Could you check a few things on this model? Use its own coordinates, in mm. A direction names the side the tool comes from. Coordinates: 2 decimals unless noted, no trailing zeros. Write each loop counter-clockwise with the first axis right and the second up, starting at its lowest first coordinate (ties: lowest second). Pieces come first, ordered by that corner, then holes. Notation, with made-up numbers: M 86.25,-22 L 134.25,-22 A29 cw 134.25,8 Z; hole C 66,59 d10. An arc over 180 degrees is marked long. Write item = value, one per line.
```python
from build123d import *

# Parameters (mm, degrees)
SKETCH1_R           = 2.54
BOSS_EXTRUDE1_DEPTH = 3.175


with BuildPart() as part:
    # Sketch1 → Boss-Extrude1 (new body)
    with BuildSketch(Plane.XY):
        with BuildLine():
            Line((-9.982299112, -2.937462922), (-4.078000987, -12.791080219))
            ThreePointArc((-4.078000987, -12.791080219), (-3.40491243, -14.361697822), (-3.175, -16.05492791))
            Line((-3.175, -16.05492791), (-3.175, -35.993911504))
            Line((-3.175, -35.993911504), (3.175, -35.993911504))
            Line((3.175, -35.993911504), (3.175, -16.05492791))
            ThreePointArc((3.175, -16.05492791), (3.40491243, -14.361697822), (4.078000987, -12.791080219))
            Line((4.078000987, -12.791080219), (9.982299112, -2.937462922))
            ThreePointArc((9.982299112, -2.937462922), (8.865013598, 4.281926793), (1.563076923, 4.504717202))
            ThreePointArc((1.563076923, 4.504717202), (0, 3.966813736), (-1.563076923, 4.504717202))
            ThreePointArc((-1.563076923, 4.504717202), (-8.865013598, 4.281926793), (-9.982299112, -2.937462922))
        make_face()
        with Locations((5.08, 0)):
            Circle(SKETCH1_R, mode=Mode.SUBTRACT)
        with Locations((-5.08, 0)):
            Circle(SKETCH1_R, mode=Mode.SUBTRACT)
    extrude(amount=BOSS_EXTRUDE1_DEPTH)


solid = part.part
```
Item 1: Imagine slicing it at B-B (z = 2.1). Write out the boundary of the cut face in (x, y) (3 decimals), and give its area (3 significant figures).
Numbers:
outline = M -9.982,-2.937 L -4.078,-12.791 A6.35 cw -3.175,-16.055 L -3.175,-35.994 L 3.175,-35.994 L 3.175,-16.055 A6.35 cw 4.078,-12.791 L 9.982,-2.937 A5.715 ccw 1.563,4.505 A2.54 cw -1.563,4.505 A5.715 ccw Z; hole C -5.08,0 d5.08; hole C 5.08,0 d5.08
area = 411 mm²
Item 2: Imagine slicing it at C-C (x = -5.08). Write out the boundary of the cut face in (y, z) (3 decimals), and give its area (3 significant figures).
Numbers:
outline = M -11.119,0 L -2.54,0 L -2.54,3.175 L -11.119,3.175 Z; M 2.54,0 L 5.715,0 L 5.715,3.175 L 2.54,3.175 Z
area = 37.3 mm²
Item 3: Imagine slicing it at A-A (y = 0). Write out the boundary of the cut face in (x, z) (3 decimals), and give its area (3 significant figures).
Numbers:
outline = M -10.795,0 L -7.62,0 L -7.62,3.175 L -10.795,3.175 Z; M -2.54,0 L 2.54,0 L 2.54,3.175 L -2.54,3.175 Z; M 7.62,0 L 10.795,0 L 10.795,3.175 L 7.62,3.175 Z
area = 36.3 mm²
Item 4: If we mould it in two halves opening along X, with no side actions, what happens to faces 4 (the face through (0, -35.994, 2)), 5 (the face through (8.947, 4.208, 1.565)), 6 (the face through (-3.41, -14.34, 1.57))? For each: pulls with the +X half, pulls with the -X half, needs draft (parallel to the pull), parting line crosses it, or undercut.
Numbers:
face_4 = needs draft
face_5 = undercut
face_6 = pulls with the -X half
Item 5: Imagine slicing it at D-D (y = -18). Write out the boundary of the cut face in (x, z) (3 decimals).
Numbers:
outline = M -3.175,0 L 3.175,0 L 3.175,3.175 L -3.175,3.175 Z
Item 6: For faces 1 (the face through (-3.175, -26, 2)), 2 (the face through (0.024, 3.967, 1.565)), 3 (the face through (3.175, -26, 2)), which set-ups out of +Z, -Z, +X, -X, +Y, -Y let a thin tool reach every point of the face, with its end or its side?
Numbers:
face_1 = +Z, -Z, -X, -Y
face_2 = +Z, -Z, +Y
face_3 = +Z, -Z, +X, -Y
Item 7: I'm going to push flat-ended pins straight in: P1, Ø4, axis at x = 5.08, y = 0, coming from the -Z side; P2, Ø1, axis at y = -29, z = 2, coming from the -X side (3 decimals); P3, Ø1, axis at x = 6, z = 1.5, coming from the -Y side; P4, Ø1.6, axis at y = -24, z = 1.5, coming from the +X side (3 decimals). Where does each tip first touch, or does it pass through?
Numbers:
P1 = through
P2 = -3.175
P3 = -10.42
P4 = 3.175
Item 8: If I drill on line 1 along Y through (x, z) = (4, 1.95); line 2 along X through (y, z) = (-33, 1.5) (3 decimals); line 3 along Y through (x, z) = (-5.08, 2) (3 decimals), over which ranges is the centre line in solid material (lowest first)?
Numbers:
line_1 = -12.92 to -2.3, 2.3 to 5.61
line_2 = -3.175 to 3.175
line_3 = -11.119 to -2.54, 2.54 to 5.715
